The model under review builds one solid part; all positions refer to its coordinate system, in mm. A direction names the side the tool comes from. Round coordinates to 2 decimals unless told otherwise and drop trailing zeros. Order: outer loops, then holes, each group sorted by start corner. A loop starts at its lowest first (then second) coordinate and runs counter-clockwise, first axis right, second up.
1) Consider section C-C (z = 516). Give the boundary of the cut face in (x, y), then the cut area to 3 significant figures.
2) Machinability: for faces 1 (the face through (-614.713, -446.165, 221.333)), 2 (the face through (56, -834, 0)), 3 (the face through (-624.657, -207, -89)), 4 (the face through (59, -1209, 250)), which of the approach directions +Z, -Z, +X, -X, +Y, -Y give a long, thin tool a straight path to every point of the face, cutting with its end or side? Answer none if there is none.
3) Consider section D-D (y = -197). Give the boundary of the cut face in (x, z).
4) Consider section B-B (x = 124.5). Give the boundary of the cut face in (y, z), then the cut area to 3 significant figures.
5) Clearance check with flat-ended pins moving along their axes: P1, Ø6, axis at y = -1104.5, z = 3, coming from the +X side; P2, Ø4, axis at y = -715, z = 388.5, coming from the -X side; P3, Ø4, axis at x = -315.5, z = 99, coming from the -Y side. State where each tip first meets the part, or that it passes through.
6) Mouldability with a two-part tool opening along X and no side actions: class faces 5 (the face through (59, -905, 127)), 6 (the face through (73.5, -40.6, 580.3)), 7 (the face through (-359.657, -1209, 123)), 8 (the face through (786.18, -1200.8, 574.65)) as pulls with the +X half, pulls with the -X half, needs draft (parallel to the pull), parting line crosses it, or undercut.
7) To check wall thickness, follow L1, parallel to X at y = -80, z = 297; L2, parallel to Z at x = 635.5, y = -606; L3, parallel to Z at x = 280, y = -1064. State the ranges of each line that lie inside material, in increasing order.
8) Consider section A-A (y = -1106). Give the boundary of the cut face in (x, z), then the cut area to 3 significant figures.
from build123d import *

# Parameters (mm, degrees)
F1_DEPTH      = 1505
F3_DEPTH      = 734.6581049648
F3_DEPTH_BACK = 865.3438950352
F5_DEPTH      = 600.001
F6_W          = 850
F6_H          = 250
F7_DEPTH      = 600
F9_DEPTH      = 905
F10_W         = 1380
F10_H         = 175
F11_DEPTH     = 420


with BuildPart() as f1:
    # F0 (on Front) → F1 (new body)
    with BuildSketch(Plane.XZ):
        Polygon((-734.6571049648, 190.5255888326), (-624.6571049648, 0), (755.3428950352, 0), (865.3428950352, 190.5255888326), (845.3428950352, 550), (725.3428950352, 600), (-594.6571049648, 600), (-714.6571049648, 550), align=None)
    extrude(amount=F1_DEPTH)

    # F2 (on Right) → F3 (cut, two sides)
    with BuildSketch(Plane.YZ) as f3_sk:
        Polygon((0, 600), (-80, 600), (0, 560), align=None)
    extrude(amount=-F3_DEPTH, mode=Mode.SUBTRACT)
    extrude(f3_sk.sketch, amount=F3_DEPTH_BACK, mode=Mode.SUBTRACT)

    # F4 (on face) → F5 (cut, through all)
    with BuildSketch(Plane.XY.offset(600)):
        Polygon((865.3428950352, 0), (825.3428950352, 0), (865.3428950352, -40), align=None)
    extrude(amount=-F5_DEPTH, mode=Mode.SUBTRACT)

    # F6 (on face) → F7 (cut)
    with BuildSketch(Plane.XZ.offset(1505)):
        with Locations((65.3428950352, 125)):
            Rectangle(F6_W, F6_H)
    extrude(amount=-F7_DEPTH, mode=Mode.SUBTRACT)

    # F8 (on face) → F9 (cut)
    with BuildSketch(Plane(origin=(0, 0, 0), x_dir=(-1, 0, 0), z_dir=(0, 1, 0))):
        Polygon((514.6571049648, 600), (514.6571049648, 560), (690.6571049648, 560), (594.6571049648, 600), align=None)
        Polygon((514.6571049648, 560), (514.6571049648, 280), (717.6104983043, 161), (734.6571049648, 190.5255888326), (714.6571049648, 550), (690.6571049648, 560), align=None)
        Polygon((-645.3428950352, 280), (-645.3428950352, 560), (-821.3428950352, 560), (-825.3428950352, 558.3333333333), (-825.3428950352, 174.4585274109), align=None)
        Polygon((-821.3428950352, 560), (-645.3428950352, 560), (-645.3428950352, 600), (-725.3428950352, 600), align=None)
        Polygon((-848.2962883747, 161), (-825.3428950352, 174.4585274109), (-825.3428950352, 558.3333333333), (-845.3428950352, 550), (-865.3428950352, 190.5255888326), align=None)
    extrude(amount=-F9_DEPTH, mode=Mode.SUBTRACT)

    # F10 (on face) → F11 (join)
    with BuildSketch(Plane(origin=(0, 0, 0), x_dir=(-1, 0, 0), z_dir=(0, 1, 0))):
        with Locations((-65.3428950352, -87.5)):
            Rectangle(F10_W, F10_H)
    extrude(amount=-F11_DEPTH)


solid = f1.part
Answer below:
1. outline: (-716.55, -1505) - (847.23, -1505) - (847.23, -905) - (645.34, -905) - (645.34, 0) - (-514.66, 0) - (-514.66, -905) - (-716.55, -905) - close
1. area: 1,990,000 mm2
2. face 1: +Z, -X, +Y
2. face 2: -Z, +X, -X, -Y
2. face 3: -Z, -X, +Y, -Y
2. face 4: -Z, -Y
3. outline: (-717.61, 161) - (-624.66, 0) - (-624.66, -175) - (755.34, -175) - (755.34, 0) - (848.3, 161) - (645.34, 280) - (645.34, 600) - (-514.66, 600) - (-514.66, 280) - close
4. outline: (-1505, 250) - (-905, 250) - (-905, 0) - (-420, 0) - (-420, -175) - (0, -175) - (0, 560) - (-80, 600) - (-1505, 600) - close
4. area: 825,000 mm2
5. P1: stops at x = 758.81
5. P2: stops at x = -514.66
5. P3: stops at y = -905
6. face 5: undercut
6. face 6: needs draft
6. face 7: undercut
6. face 8: pulls with the +X half
7. L1: x = -514.66 to 645.34
7. L2: z = 0 to 600
7. L3: z = 250 to 600
8. outline: (-734.66, 190.53) - (-624.66, 0) - (-359.66, 0) - (-359.66, 250) - (490.34, 250) - (490.34, 0) - (755.34, 0) - (865.34, 190.53) - (845.34, 550) - (725.34, 600) - (-594.66, 600) - (-714.66, 550) - close
8. area: 711,000 mm2
